The model under review builds one solid part; all positions refer to its coordinate system, in mm. Face numbers are marked on the shaded views. A direction names the side the tool comes from. Coordinates: 2 decimals unless noted, no trailing zeros. Order: outer loops, then holes, each group sorted by start corner. A loop starts at its lowest first (then second) coordinate and runs counter-clockwise, first axis right, second up.
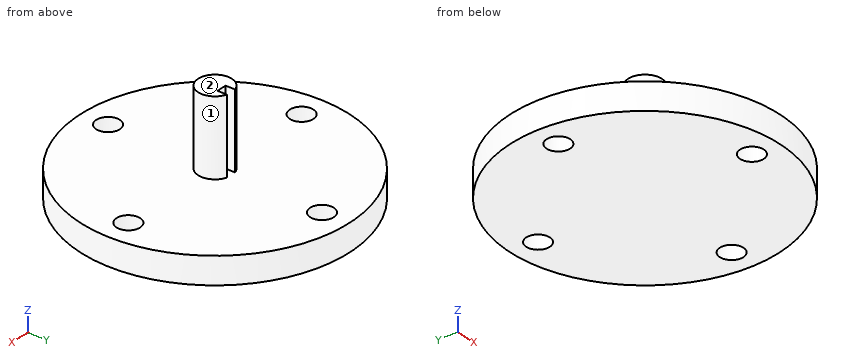
```python
from build123d import *

# Parameters (mm, degrees)
SKETCH1_R           = 63.5
SKETCH1_R_2         = 5.55625
BOSS_EXTRUDE1_DEPTH = 12.7
BOSS_EXTRUDE5_DEPTH = 48.26


with BuildPart() as part:
    # Sketch1 → Boss-Extrude1 (new body)
    with BuildSketch(Plane.XY):
        Circle(SKETCH1_R)
        with Locations((-50.8, 0)):
            Circle(SKETCH1_R_2, mode=Mode.SUBTRACT)
        with Locations((0, 50.8)):
            Circle(SKETCH1_R_2, mode=Mode.SUBTRACT)
        with Locations((50.8, 0)):
            Circle(SKETCH1_R_2, mode=Mode.SUBTRACT)
        with Locations((0, -50.8)):
            Circle(SKETCH1_R_2, mode=Mode.SUBTRACT)
    extrude(amount=BOSS_EXTRUDE1_DEPTH)

    # Sketch2 → Boss-Extrude5 (add)
    with BuildSketch(Plane(origin=(0, 0, 0), x_dir=(-1, 0, 0), z_dir=(0, 0, -1))):
        with BuildLine():
            Line((-2.413, 7.561834252), (-2.413, 3.1115))
            Line((-2.413, 3.1115), (2.413, 3.1115))
            Line((2.413, 3.1115), (2.413, 7.561834252))
            ThreePointArc((2.413, 7.561834252), (0, -7.9375), (-2.413, 7.561834252))
        make_face()
    extrude(amount=-BOSS_EXTRUDE5_DEPTH)


solid = part.part
```
(1) Wall thickness on probe 1 along Y at (x, z) = (0, 8); probe 2 along Z at (x, y) = (-19, -50); probe 3 along Y at (x, z) = (50, 8): over which ranges is each line inside the solid? List them lowest first.
A:
probe 1: y = -63.5 to -56.36, -45.24 to 45.24, 56.36 to 63.5
probe 2: z = 0 to 12.7
probe 3: y = -39.14 to -5.5, 5.5 to 39.14
(2) For pin 1 Ø6 at (y, z) = (30.5, 9.5) entering from +X; pin 2 Ø5 at (x, y) = (-40, 41) entering from +Z; pin 3 Ø4 at (x, z) = (-12.5, 8) entering from -Y, all flat-tipped, find the tip position at first contact; note any pin that passes through.
A:
pin 1: stops at x = 57.24
pin 2: stops at z = 12.7
pin 3: stops at y = -62.63
(3) Machinability: for the marked faces 1 and 2, which of the approach directions +Z, -Z, +X, -X, +Y, -Y give a long, thin tool a straight path to every point of the face, cutting with its end or side? Answer none if there is none.
A:
face 1: +Z
face 2: +Z, +X, -X, +Y, -Y
(4) We need section C-C, the plane y = -50.8. Write out the cut boundary in (x, z).
A:
outline: (-38.1, 0) - (-5.56, 0) - (-5.56, 12.7) - (-38.1, 12.7) - close; (5.56, 0) - (38.1, 0) - (38.1, 12.7) - (5.56, 12.7) - close
(5) We need section B-B, the plane x = 0. Write out the cut boundary in (y, z), and give its area (3 significant figures).
A:
outline: (-63.5, 0) - (-56.36, 0) - (-56.36, 12.7) - (-63.5, 12.7) - close; (-45.24, 0) - (45.24, 0) - (45.24, 12.7) - (3.11, 12.7) - (3.11, 48.26) - (-7.94, 48.26) - (-7.94, 12.7) - (-45.24, 12.7) - close; (56.36, 0) - (63.5, 0) - (63.5, 12.7) - (56.36, 12.7) - close
area: 1,720 mm2
(6) We need section A-A, the plane y = 0. Write out the cut boundary in (x, z), and give its area (3 significant figures).
A:
outline: (-63.5, 0) - (-56.36, 0) - (-56.36, 12.7) - (-63.5, 12.7) - close; (-45.24, 0) - (45.24, 0) - (45.24, 12.7) - (7.94, 12.7) - (7.94, 48.26) - (-7.94, 48.26) - (-7.94, 12.7) - (-45.24, 12.7) - close; (56.36, 0) - (63.5, 0) - (63.5, 12.7) - (56.36, 12.7) - close
area: 1,900 mm2
